from build123d import *

# Parameters (mm, degrees)
PAD001_DEPTH         = 5
SKETCH007_R          = 1.4
POCKET001_DEPTH      = 5.001
POCKET001_DEPTH_BACK = 0.001
POCKET002_DEPTH      = 2
SKETCH009_R          = 112.8
POCKET003_DEPTH      = 2.001


with BuildPart() as part:
    # Sketch005 → Pad001 (new body)
    with BuildSketch(Plane.XY):
        with BuildLine():
            Line((-10.529704, 0), (10.529704, 0))
            ThreePointArc((10.529704, 0), (12.060526, 0.712916), (12.5, 2.343415))
            Line((10, 16.686829), (12.5, 2.343415))
            ThreePointArc((10, 16.686829), (8.633576, 19.061643), (6.059408, 20))
            Line((-6.059408, 20), (6.059408, 20))
            ThreePointArc((-6.059408, 20), (-8.633576, 19.061643), (-10, 16.686829))
            Line((-12.5, 2.343415), (-10, 16.686829))
            ThreePointArc((-12.5, 2.343415), (-12.060526, 0.712916), (-10.529704, 0))
        make_face()
    extrude(amount=-PAD001_DEPTH)

    # Sketch007 → Pocket001 (cut, two sides)
    with BuildSketch(Plane.XY) as pocket001_sk:
        with Locations((-4.5, 16)):
            Circle(SKETCH007_R)
        with Locations((4.5, 16)):
            Circle(SKETCH007_R)
        with Locations((7.5, 4)):
            Circle(SKETCH007_R)
        with Locations((-7.5, 4)):
            Circle(SKETCH007_R)
    extrude(amount=-POCKET001_DEPTH, mode=Mode.SUBTRACT)
    extrude(pocket001_sk.sketch, amount=POCKET001_DEPTH_BACK, mode=Mode.SUBTRACT)

    # Sketch008 → Pocket002 (cut)
    with BuildSketch(Plane.XY):
        Polygon((-9.001111, 6.6), (-10.502221, 4), (-9.001111, 1.4), (-5.998889, 1.4), (-4.497779, 4), (-5.998889, 6.6), align=None)
        Polygon((9.001111, 1.4), (10.502221, 4), (9.001111, 6.6), (5.998889, 6.6), (4.497779, 4), (5.998889, 1.4), align=None)
        Polygon((6.001111, 13.4), (7.502221, 16), (6.001111, 18.6), (2.998889, 18.6), (1.497779, 16), (2.998889, 13.4), align=None)
        Polygon((-6.001111, 13.4), (-2.998889, 13.4), (-1.497779, 16), (-2.998889, 18.6), (-6.001111, 18.6), (-7.502221, 16), align=None)
    extrude(amount=-POCKET002_DEPTH, mode=Mode.SUBTRACT)

    # Sketch009 (on DatumPlane) → Pocket003 (cut, through all)
    with BuildSketch(Plane.XY.offset(-3)):
        with Locations((0, -100.8)):
            Circle(SKETCH009_R)
    extrude(amount=-POCKET003_DEPTH, mode=Mode.SUBTRACT)


solid = part.part
Model file for the job. Use its own axes, mm. A direction names the side the tool comes from. Give positions to 0.01 mm unless a question says otherwise; leave off trailing zeros. Order: outer loops, then holes, each group sorted by start corner. A loop starts at its lowest first (then second) coordinate and runs counter-clockwise, first axis right, second up. Notation, with made-up numbers: (83.5, 65) - (93.5, 65) arc R18 ccw to (93.5, 88) - close; hole circle Ø9 at (66, 14.5). An arc over 180 degrees is marked (long way). One line per item, written item: value.
Item 1: Slice it at B-B (x = -6.5). List the corners of the cut face in (y, z).
Response values:
outline: (0, -3) - (3.02, -3) - (3.02, -2) - (1.4, -2) - (1.4, 0) - (0, 0) - close; (4.98, -3) - (11.81, -3) - (11.81, -5) - (19.98, -5) - (19.98, 0) - (17.74, 0) - (17.74, -2) - (14.26, -2) - (14.26, 0) - (6.6, 0) - (6.6, -2) - (4.98, -2) - close
Item 2: Slice it at D-D (z = -0.6). Give the number of separate pieces and of enclosed holes in the cut face, then the cut area to 3 significant figures.
Response values:
separate pieces: 1
enclosed holes: 4
area: 346 mm2
Item 3: Slice it at C-C (y = 4.75). List the corners of the cut face in (x, z), then the cut area to 3 significant figures.
Response values:
outline: (-12.08, -3) - (-8.68, -3) - (-8.68, -2) - (-10.07, -2) - (-10.07, 0) - (-12.08, 0) - close; (-6.32, -3) - (6.32, -3) - (6.32, -2) - (4.93, -2) - (4.93, 0) - (-4.93, 0) - (-4.93, -2) - (-6.32, -2) - close; (8.68, -3) - (12.08, -3) - (12.08, 0) - (10.07, 0) - (10.07, -2) - (8.68, -2) - close
area: 47.2 mm2
Item 4: Two-plate mould, pull along Y, no slides. Class faces 4 (the flat face through (-2.26, 14.68, -0.99)), 5 (the flat face through (0, 6, -3)), 6 (the cylindrical face through (-8.6, 19.09, -2.46)), 7 (the cylindrical face through (5.25, 17.18, -3.48)): released by +Y, released by -Y, zero draft, split by the parting line, or undercut.
Response values:
face 4: undercut
face 5: zero draft
face 6: released by +Y
face 7: undercut
Item 5: Pin check, flat tips, straight feed: pin 1 Ø4 at (x, y) = (8, 4) entering from +Z; pin 2 Ø3 at (y, z) = (7, -1.5) entering from +X; pin 3 Ø1 at (x, z) = (-7, -1) entering from +Y. Stop position of each tip, or through.
Response values:
pin 1: z = -2
pin 2: x = 11.95
pin 3: y = 19.98
Item 6: Slice it at A-A (z = -3.6). List the corners of the cut face in (x, y).
Response values:
outline: (-10.91, 11.47) arc R112.8 cw to (10.91, 11.47) - (10, 16.69) arc R4 ccw to (6.06, 20) - (-6.06, 20) arc R4 ccw to (-10, 16.69) - close; hole circle Ø2.8 at (-4.5, 16); hole circle Ø2.8 at (4.5, 16)
Item 7: Wall check: line 1 (Y direction, x = 4.5, z = -2.95); line 2 (X direction, y = 1.75, z = -1.65); line 3 (X direction, y = 17.25, z = -3.25). Give the ranges that are in metal, low to high.
Response values:
line 1: 0 to 14.6, 17.4 to 20
line 2: -12.51 to -9.2, -5.8 to 5.8, 9.2 to 12.51
line 3: -9.86 to -5.13, -3.87 to 3.87, 5.13 to 9.86
Item 8: Tool access for faces 1 (the flat face through (-3, 15, -2)), 2 (the cylindrical face through (0, 12, -4)), 3 (the flat face through (0, 0, -1)): list every direction of +Z, -Z, +X, -X, +Y, -Y with a clear straight run to the whole face (end or side of a thin tool).
Response values:
face 1: +Z
face 2: -Z, -Y
face 3: +Z, -Z, +X, -X, -Y
